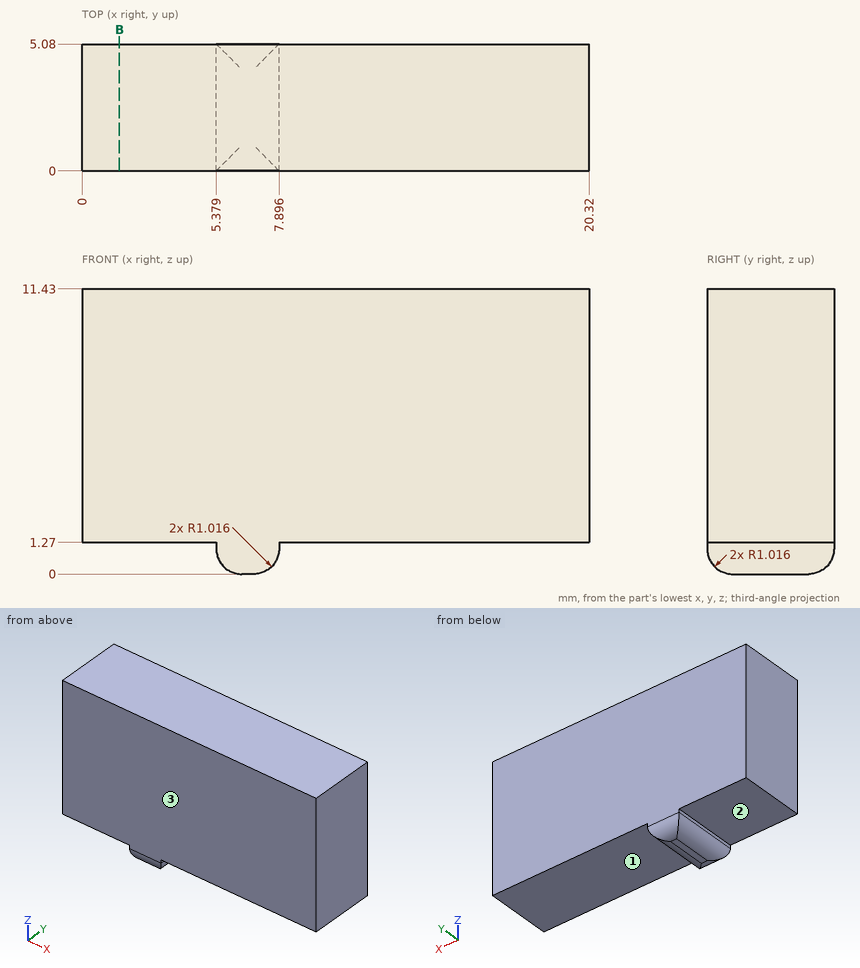
Could you check a few things on this drawing? It's one solid part, dimensions in mm from its lowest x, y, z. A direction names the side the tool comes from. Give positions to 0.01 mm unless a question says otherwise; leave off trailing zeros. Order: outer loops, then holes, each group sorted by start corner. A loop starts at its lowest first (then second) coordinate and runs counter-clockwise, first axis right, second up. Notation, with made-up numbers: (50.25, 7.5) - (78.25, 7.5) arc R21 cw to (78.25, 21.5) - close; hole circle Ø1 at (51, -4). An arc over 180 degrees is marked (long way). Return JSON: item names as keys, results as strings. Group by question number.
Q1. Please list where these lines run through material, in increasing order: line 1 along Z through (x, y) = (13.75, 1.8); line 2 along Z through (x, y) = (6, 3.8). Write a range as [from, to].
Q2. Suppose I cut it at B-B, the plane x = 1.5. Please give me the cut outline in (y, z).
Q3. Which directions (+Z, -Z, +X, -X, +Y, -Y) give clear straight access to the entire face, cutting with the end or side of a thin tool? Please do the marked faces 1, 2 and 3.
Q4. Will this pin go through, and if not, where does the flat tip stop? pin 1 Ø3 at (x, y) = (2.5, 2.5) entering from -Z.
Resolved:
{
 "1": {"line 1": "z = [1.27, 11.43]", "line 2": "z = [0.08, 11.43]"},
 "2": {"outline": "(0, 1.27) - (5.08, 1.27) - (5.08, 11.43) - (0, 11.43) - close"},
 "3": {"face 1": "-Z, +X, +Y, -Y", "face 2": "-Z, -X, +Y, -Y", "face 3": "+Z, -Z, +X, -X, -Y"},
 "4": {"pin 1": "stops at z = 1.27"}
}
